from build123d import *

# Parameters (mm, degrees)
BOSS_EXTRUDE1_DEPTH = 15
CUT_EXTRUDE1_DEPTH  = 10
SKETCH4_R           = 15
SKETCH4_R_2         = 1.6
CUT_EXTRUDE2_DEPTH  = 10
BOSS_EXTRUDE2_DEPTH = 10
BOSS_EXTRUDE3_DEPTH = 10
SKETCH7_R           = 2.6
CUT_EXTRUDE3_DEPTH  = 10
SKETCH8_R           = 2.6
CUT_EXTRUDE4_DEPTH  = 10


with BuildPart() as part:
    # Sketch1 → Boss-Extrude1 (new body)
    with BuildSketch(Plane(origin=(0, 0, 0), x_dir=(1, 0, 0), z_dir=(0, 1, 0))):
        with BuildLine():
            Line((-33.262289521, -33.262289521), (-132.330467636, -33.262289521))
            Line((-132.330467636, -33.262289521), (-132.330467636, -19.482767229))
            ThreePointArc((-132.330467636, -19.482767229), (-130.821698058, -14.200816273), (-126.750666454, -10.512714699))
            Line((-126.750666454, -10.512714699), (-37.682488339, 33.377669927))
            ThreePointArc((-37.682488339, 33.377669927), (-35.531592794, 34.146727348), (-33.262289521, 34.407617396))
            Line((-33.262289521, 34.407617396), (24.407617396, 34.407617396))
            ThreePointArc((24.407617396, 34.407617396), (31.478685208, 31.478685208), (34.407617396, 24.407617396))
            Line((34.407617396, 24.407617396), (34.407617396, -33.262289521))
            Line((34.407617396, -33.262289521), (-33.262289521, -33.262289521))
        make_face()
        with BuildLine():
            Line((-31.892027887, 10.478694381), (-98.33678925, -22.263483514))
            ThreePointArc((-98.33678925, -22.263483514), (-102.487767169, -20.853028863), (-101.077312518, -16.702050945))
            Line((-101.077312518, -16.702050945), (-34.632551154, 16.04012695))
            ThreePointArc((-34.632551154, 16.04012695), (-30.481573236, 14.629672299), (-31.892027887, 10.478694381))
        make_face(mode=Mode.SUBTRACT)
        with BuildLine():
            Line((-123.700729269, -16.702050945), (-34.632551154, 27.188333681))
            ThreePointArc((-34.632551154, 27.188333681), (-30.481573236, 25.77787903), (-31.892027887, 21.626901112))
            Line((-31.892027887, 21.626901112), (-120.960206002, -22.263483514))
            ThreePointArc((-120.960206002, -22.263483514), (-125.11118392, -20.853028863), (-123.700729269, -16.702050945))
        make_face(mode=Mode.SUBTRACT)
        with BuildLine():
            Line((-78.371246836, -16.869773094), (-34.549902224, 4.72419807))
            ThreePointArc((-34.549902224, 4.72419807), (-30.649295385, 3.398816638), (-31.974676817, -0.501790201))
            Line((-31.974676817, -0.501790201), (-75.796021429, -22.095761365))
            ThreePointArc((-75.796021429, -22.095761365), (-79.696628268, -20.770379933), (-78.371246836, -16.869773094))
        make_face(mode=Mode.SUBTRACT)
    extrude(amount=BOSS_EXTRUDE1_DEPTH)

    # Sketch2 → Cut-Extrude1 (cut)
    with BuildSketch(Plane(origin=(0, 15, 0), x_dir=(1, 0, 0), z_dir=(0, 1, 0))):
        Polygon((-17.714466094, 21.25), (-21.25, 17.714466094), (-21.25, -17.714466094), (-17.714466094, -21.25), (17.714466094, -21.25), (21.25, -17.714466094), (21.25, 17.714466094), (17.714466094, 21.25), align=None)
    extrude(amount=-CUT_EXTRUDE1_DEPTH, mode=Mode.SUBTRACT)

    # Sketch4 → Cut-Extrude2 (cut)
    with BuildSketch(Plane(origin=(0, 5, 0), x_dir=(1, 0, 0), z_dir=(0, 1, 0))):
        with Locations(Location((0, 0, 0), (0, 0, 270))):
            Circle(SKETCH4_R)
        with Locations(Location((-15.25, -15.25, 0), (0, 0, 270))):
            Circle(SKETCH4_R_2)
        with Locations(Location((-15.25, 15.25, 0), (0, 0, 270))):
            Circle(SKETCH4_R_2)
        with Locations(Location((15.25, 15.25, 0), (0, 0, 270))):
            Circle(SKETCH4_R_2)
        with Locations(Location((15.25, -15.25, 0), (0, 0, 270))):
            Circle(SKETCH4_R_2)
    extrude(amount=-CUT_EXTRUDE2_DEPTH, mode=Mode.SUBTRACT)

    # Sketch5 → Boss-Extrude2 (add)
    with BuildSketch(Plane.XY.offset(33.262289521)):
        with BuildLine():
            Line((-132.330467636, 15), (-132.330467636, 29.515702772))
            ThreePointArc((-132.330467636, 29.515702772), (-131.098434148, 34.324316216), (-127.705914986, 37.9480551))
            Line((-127.705914986, 37.9480551), (-37.989603896, 95.140317474))
            ThreePointArc((-37.989603896, 95.140317474), (-35.41384195, 96.308056898), (-32.614156546, 96.707965146))
            Line((-32.614156546, 96.707965146), (24.407617396, 96.707965146))
            ThreePointArc((24.407617396, 96.707965146), (31.478685208, 93.779032958), (34.407617396, 86.707965146))
            Line((34.407617396, 86.707965146), (34.407617396, 15))
            Line((34.407617396, 15), (-132.330467636, 15))
        make_face()
    extrude(amount=-BOSS_EXTRUDE2_DEPTH)

    # Sketch6 → Boss-Extrude3 (add)
    with BuildSketch(Plane(origin=(34.407617396, 0, 0), x_dir=(0, 0, -1), z_dir=(1, 0, 0))):
        Polygon((-23.262289521, 86.707965146), (24.407617396, 15), (-23.262289521, 15), align=None)
    extrude(amount=-BOSS_EXTRUDE3_DEPTH)

    # Sketch7 → Cut-Extrude3 (cut)
    with BuildSketch(Plane(origin=(0, 0, 23.262289521), x_dir=(-1, 0, 0), z_dir=(0, 0, -1))):
        with Locations((-13.732807518, 76.033155267)):
            Circle(SKETCH7_R)
        with Locations((33.101778739, 29.198569011)):
            Circle(SKETCH7_R)
        with Locations((33.101778739, 76.033155267)):
            Circle(SKETCH7_R)
        with Locations((-13.732807518, 29.198569011)):
            Circle(SKETCH7_R)
        with Locations((118.329007759, 29.198569011)):
            Circle(SKETCH7_R)
        with Locations((77.104397796, 29.198569011)):
            Circle(SKETCH7_R)
        with Locations((77.104397796, 49.667805409)):
            Circle(SKETCH7_R)
    extrude(amount=-CUT_EXTRUDE3_DEPTH, mode=Mode.SUBTRACT)

    # Sketch8 → Cut-Extrude4 (cut)
    with BuildSketch(Plane.ZY.offset(-24.407617396)):
        with Locations((15.467402897, 24.417657132)):
            Circle(SKETCH8_R)
        with Locations((15.467402897, 60.531845861)):
            Circle(SKETCH8_R)
        with Locations((-8.540529995, 24.417657132)):
            Circle(SKETCH8_R)
    extrude(amount=-CUT_EXTRUDE4_DEPTH, mode=Mode.SUBTRACT)


solid = part.part
Here's how the part is built. I have some questions about the finished solid (model axes, mm). A direction names the side the tool comes from. Coordinates: 2 decimals unless noted, no trailing zeros. Write each loop counter-clockwise with the first axis right and the second up, starting at its lowest first coordinate (ties: lowest second). Pieces come first, ordered by that corner, then holes.
Item 1: On a 3-axis mill with a long thin cutter (end or side, diameter ignored), from which of +Z, -Z, +X, -X, +Y, -Y can I reach the whole of each face in a straight line? I mean faces 4 (the flat face through (-19.457, 10.07, -19.507)), 5 (the flat face through (-68.32, 7.4, 0.56)), 6 (the flat face through (-48, 15, -12)). Say none if no direction works.
Item 2: If we mould it in two halves opening along Z, with no side actions, what happens to faces 1 (the cylindrical face through (-131.132, 34.263, 28.332)), 2 (the flat face through (-21.25, 10, 0)), 3 (the flat face through (-48, 47, 23.262))? For each: +Z half, -Z half, draft (parallel to the pull), parting line (faces both ways), or undercut.
Item 3: Will these pins go through, and if not, where does the flat tip stop? pin 1 (4.5 mm diameter, centred on x = -77.1, y = 49.67, fed in from -Z); pin 2 (10 mm diameter, centred on y = 72.5, z = 10, fed in from -X); pin 3 (4 mm diameter, centred on x = -13.5, z = 7, fed in from +Y); pin 4 (5 mm diameter, centred on y = 10.5, z = -6.5, fed in from -X).
Item 4: I want a section at C-C on y = 83.5. Write out the boundary of the cut face in (x, z), and give its area (3 significant figures).
Item 5: If I drill on line 1 (X direction, y = 1, z = 0); line 2 (Z direction, x = 14, y = 5.5); line 3 (Z direction, x = -99.5, y = 52), over which ranges is the centre line in solid material (lowest first)?
Item 6: I want a section at A-A on x = 0. Write out the boundary of the cut face in (y, z).
Item 7: I want a section at B-B on x = -40.5. Write out the boundary of the cut face in (y, z).
Findings below:
1. face 4: +Y
1. face 5: +Y, -Y
1. face 6: -Z, -X, +Y
2. face 1: draft
2. face 2: undercut
2. face 3: -Z half
3. pin 1: passes through
3. pin 2: stops at x = 24.41
3. pin 3: stops at y = 5
3. pin 4: stops at x = -97.3
4. outline: (-56.25, 23.26) - (24.41, 23.26) - (24.41, 21.13) - (34.41, 21.13) - (34.41, 33.26) - (-56.25, 33.26) - close
4. area: 928 mm2
5. line 1: x = -105.42 to -89.81, -75.78 to -67.18, -53.16 to -44.14, -31.26 to -15, 15 to 34.41
5. line 2: z = -34.41 to -21.25, 21.25 to 33.26
5. line 3: z = 23.26 to 33.26
6. outline: (0, -34.41) - (15, -34.41) - (15, -21.25) - (5, -21.25) - (5, -15) - (0, -15) - close; (0, 15) - (5, 15) - (5, 21.25) - (15, 21.25) - (15, 23.26) - (96.71, 23.26) - (96.71, 33.26) - (0, 33.26) - close
7. outline: (0, -31.99) - (15, -31.99) - (15, -24.3) - (0, -24.3) - close; (0, -17.39) - (15, -17.39) - (15, -13.15) - (0, -13.15) - close; (0, -6.24) - (15, -6.24) - (15, -1.79) - (0, -1.79) - close; (0, 4.7) - (15, 4.7) - (15, 23.26) - (93.54, 23.26) - (93.54, 33.26) - (0, 33.26) - close
